from build123d import *

# Parameters (mm, degrees)
ESBO_O1_W                                      = 130
ESBO_O1_H                                      = 20
RESSALTO_EXTRUS_O1_DEPTH                       = 95
CORTE_EXTRUS_O2_REACH                          = 22
CORTE_EXTRUS_O3_DEPTH                          = 1
CORTE_EXTRUS_O3_DEPTH_BACK                     = 131
BROCA_DE_ROSQUEAR_DE_CANO_PARA_TARRAXA_D_D     = 6.579997
BROCA_DE_ROSQUEAR_DE_CANO_PARA_TARRAXA_D_DEPTH = 10
BROCA_DE_ROSQUEAR_DE_CANO_PARA_TARRAXA_D_TIP   = 1.976830535
BROCA_DE_ROSQUEAR_DE_CANO_PARA_TARRA_2_D       = 6.579997
BROCA_DE_ROSQUEAR_DE_CANO_PARA_TARRA_2_DEPTH   = 10
BROCA_DE_ROSQUEAR_DE_CANO_PARA_TARRA_2_TIP     = 1.976830535
FILETE2_R                                      = 5
CORTE_EXTRUS_O5_DEPTH                          = 131
RESSALTO_EXTRUS_O2_REACH                       = 57.5
ESBO_O15_W                                     = 28.25
ESBO_O15_H                                     = 8.1
ESBO_O16_W                                     = 50
ESBO_O16_H                                     = 2
CORTE_EXTRUS_O6_DEPTH                          = 40.5
CORTE_EXTRUS_O7_REACH                          = 21.612
ESBO_O17_W                                     = 55
ESBO_O17_H                                     = 19.621819015


with BuildPart() as part:
    # Esboço1 → Ressalto-extrusão1 (new body)
    with BuildSketch(Plane.XY):
        Rectangle(ESBO_O1_W, ESBO_O1_H)
    extrude(amount=RESSALTO_EXTRUS_O1_DEPTH)

    # Esboço2 → Corte-extrusão2 (cut, up to next)
    with BuildSketch(Plane(origin=(0, 10, 0), x_dir=(1, 0, 0), z_dir=(0, 1, 0)), mode=Mode.PRIVATE) as corte_extrus_o2_sk1:
        with BuildLine():
            Line((15, 0), (-65, 0))
            Line((-65, 0), (-65, -80))
            Line((-65, -80), (-30.4, -80))
            ThreePointArc((-30.4, -80), (7.930824636, -69.206398281), (35, -40))
            Line((35, -40), (15, 0))
        make_face()
    corte_extrus_o2_tool1 = extrude(corte_extrus_o2_sk1.sketch, amount=-CORTE_EXTRUS_O2_REACH, mode=Mode.PRIVATE) & part.part
    add(corte_extrus_o2_tool1.solids().sort_by_distance((-21.312918, 10, 38.404489))[0], mode=Mode.SUBTRACT)

    # Esboço3 → Corte-extrusão3 (cut, two sides)
    with BuildSketch(Plane(origin=(65, 0, 0), x_dir=(0, 0, -1), z_dir=(1, 0, 0))) as corte_extrus_o3_sk:
        Polygon((200.200134404, 50.040026881), (0, 10), (-95, -9), (-295.200134404, -49.040026881), (-375.280188165, 351.360241926), (120.120080642, 450.440295688), align=None)
    extrude(amount=CORTE_EXTRUS_O3_DEPTH, mode=Mode.SUBTRACT)
    extrude(corte_extrus_o3_sk.sketch, amount=-CORTE_EXTRUS_O3_DEPTH_BACK, mode=Mode.SUBTRACT)

    # Broca de rosquear de cano para tarraxa d
    with Locations(Plane(origin=(65, 0, 0), x_dir=(0, 0, -1), z_dir=(1, 0, 0))):
        with Locations((-20, -1.945)):
            Hole(BROCA_DE_ROSQUEAR_DE_CANO_PARA_TARRAXA_D_D / 2, depth=BROCA_DE_ROSQUEAR_DE_CANO_PARA_TARRAXA_D_DEPTH)
            with Locations((0, 0, -(BROCA_DE_ROSQUEAR_DE_CANO_PARA_TARRAXA_D_DEPTH + BROCA_DE_ROSQUEAR_DE_CANO_PARA_TARRAXA_D_TIP / 2))):  # 118° drill point
                Cone(0, BROCA_DE_ROSQUEAR_DE_CANO_PARA_TARRAXA_D_D / 2, BROCA_DE_ROSQUEAR_DE_CANO_PARA_TARRAXA_D_TIP, mode=Mode.SUBTRACT)

    # Broca de rosquear de cano para tarra 2
    with Locations(Plane(origin=(12, 0, -6), x_dir=(0.447213595, 0, 0.894427191), z_dir=(-0.894427191, 0, 0.447213595))):
        with Locations((26.708203932, -1.945)):
            Hole(BROCA_DE_ROSQUEAR_DE_CANO_PARA_TARRA_2_D / 2, depth=BROCA_DE_ROSQUEAR_DE_CANO_PARA_TARRA_2_DEPTH)
            with Locations((0, 0, -(BROCA_DE_ROSQUEAR_DE_CANO_PARA_TARRA_2_DEPTH + BROCA_DE_ROSQUEAR_DE_CANO_PARA_TARRA_2_TIP / 2))):  # 118° drill point
                Cone(0, BROCA_DE_ROSQUEAR_DE_CANO_PARA_TARRA_2_D / 2, BROCA_DE_ROSQUEAR_DE_CANO_PARA_TARRA_2_TIP, mode=Mode.SUBTRACT)

    # Filete2
    filete2_edges = [part.edges().sort_by_distance(p)[0] for p in [
        (65, -9.5, 95),
    ]]
    fillet(filete2_edges, radius=FILETE2_R)

    # Esboço14 → Corte-extrusão5 (cut, through all)
    with BuildSketch(Plane(origin=(65, 0, 0), x_dir=(0, 0, -1), z_dir=(1, 0, 0))):
        Polygon((-40.5, -10), (-39.5, -10), (-39.5, 2.1), (-40.5, 1.9), align=None)
    extrude(amount=-CORTE_EXTRUS_O5_DEPTH, mode=Mode.SUBTRACT)

    # Esboço15 → Ressalto-extrusão2 (add, up to next)
    with BuildSketch(Plane.XY.offset(39.5), mode=Mode.PRIVATE) as ressalto_extrus_o2_sk1:
        with Locations((49.875, -2.95)):
            Rectangle(ESBO_O15_W, ESBO_O15_H)
    ressalto_extrus_o2_tool1 = extrude(ressalto_extrus_o2_sk1.sketch, amount=RESSALTO_EXTRUS_O2_REACH, mode=Mode.PRIVATE) - part.part
    add(ressalto_extrus_o2_tool1.solids().sort_by_distance((49.875, -2.95, 39.5))[0])

    # Esboço16 → Corte-extrusão6 (cut)
    with BuildSketch(Plane(origin=(0, 0, 0), x_dir=(-1, 0, 0), z_dir=(0, 0, -1))):
        with Locations((-40, -9)):
            Rectangle(ESBO_O16_W, ESBO_O16_H)
    extrude(amount=-CORTE_EXTRUS_O6_DEPTH, mode=Mode.SUBTRACT)

    # Esboço17 → Corte-extrusão7 (cut, up to next)
    with BuildSketch(Plane(origin=(0, 9.615384615, 1.923076923), x_dir=(1, 0, 0), z_dir=(0, 0.980580676, 0.196116135)), mode=Mode.PRIVATE) as corte_extrus_o7_sk1:
        with Locations((-37.5, -86.4868795)):
            Rectangle(ESBO_O17_W, ESBO_O17_H)
    corte_extrus_o7_tool1 = extrude(corte_extrus_o7_sk1.sketch, amount=-CORTE_EXTRUS_O7_REACH, mode=Mode.PRIVATE) & part.part
    add(corte_extrus_o7_tool1.solids().sort_by_distance((-37.5, -7.346088, 86.73044))[0], mode=Mode.SUBTRACT)


solid = part.part
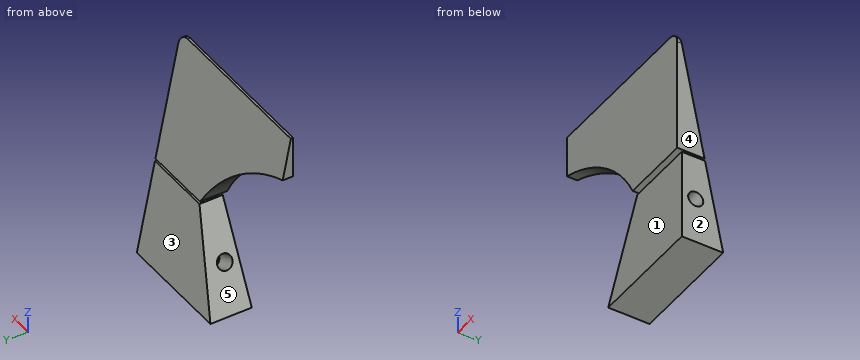
Here's how the part is built. I have some questions about the finished solid (model axes, mm). Face numbers are marked on the shaded views. A direction names the side the tool comes from. Round coordinates to 2 decimals unless told otherwise and drop trailing zeros. Write each loop counter-clockwise with the first axis right and the second up, starting at its lowest first coordinate (ties: lowest second). Pieces come first, ordered by that corner, then holes.
1. If we mould it in two halves opening along Z, with no side actions, what happens to the marked faces 3, 4 and 5? For each: released by +Z, released by -Z, zero draft, split by the parting line, or undercut.
2. I need wall thicknesses on L1, parallel to Y at x = 62, z = 20 (3 decimals); L2, parallel to Y at x = 30.5, z = 30; L3, parallel to X at y = -4.5, z = 60.5. Which ranges of each line are inside material? Lowest first, please.
3. Suppose I cut it at A-A (x = 18). List the corners of the cut face in (y, z) for me, and give its area (3 significant figures).
4. For the marked faces 1 and 2, which set-ups out of +Z, -Z, +X, -X, +Y, -Y let a thin tool reach every point of the face, with its end or its side?
5. Will these pins go through, and if not, where does the flat tip stop? pin 1 Ø1 at (x, z) = (6, 76) entering from +Y; pin 2 Ø0.5 at (y, z) = (-3.5, 40) entering from -X; pin 3 Ø3 at (y, z) = (4, 40) entering from +X; pin 4 Ø0.8 at (y, z) = (-5, 40) entering from +X.
6. Suppose I cut it at D-D (y = 3.75). List the corners of the cut face in (x, z) for me (3 decimals).
7. Suppose I cut it at C-C (z = 82.5). List the corners of the cut face in (x, y) for me, and give its area (4 significant figures).
8. Suppose I cut it at B-B (x = 41.5). List the corners of the cut face in (y, z) for me.
Answer sheet:
1. face 3: released by +Z
1. face 4: zero draft
1. face 5: undercut
2. L1: y = -8 to -5.235, 1.345 to 6
2. L2: y = -8 to 4
2. L3: x = 19.45 to 65
3. outline: (-10, 61.8) - (-2.36, 61.8) - (-9, 95) - (-10, 95) - close; (-8, 0) - (10, 0) - (8.8, 6) - (-8, 6) - close
3. area: 248 mm2
4. face 1: -Z, +X, -X, -Y
4. face 2: +Z, -Z, +X, +Y, -Y
5. pin 1: stops at y = -5.1
5. pin 2: stops at x = 35.75
5. pin 3: passes through
5. pin 4: stops at x = 64
6. outline: (15, 0) - (65, 0) - (65, 31.25) - (30.625, 31.25) - close
7. outline: (-10, -10) - (65, -10) - (65, -6.5) - (-10, -6.5) - close
7. area: 262.5 mm2
8. outline: (-10, 40.5) - (-7, 40.5) - (-7, 39.5) - (-8, 39.5) - (-8, 0) - (10, 0) - (2.1, 39.5) - (1.1, 39.5) - (1.1, 40.5) - (1.9, 40.5) - (-9, 95) - (-10, 95) - close
